Geometry: final body of the model. Coordinates: model frame, mm. A direction names the side the tool comes from. Coordinates: 2 decimals unless noted, no trailing zeros. Order: outer loops, then holes, each group sorted by start corner. A loop starts at its lowest first (then second) coordinate and runs counter-clockwise, first axis right, second up. Notation, with made-up numbers: M -0.5,-33 L 43.5,-33 A28 cw 43.5,-9 Z; hole C 50.5,64 d8. An arc over 180 degrees is marked long. Use CSV: the item, a comma, the result in double quotes. Start each with the question number.
Q1. Section query A-A, the plane y = 1.4. Output: boundary loops of the cut face in (x, z).
Q2. Ray query, probe 1 along X at (y, z) = (0.1, 3.75); probe 2 along Z at (x, y) = (6.5, 0.7); probe 3 along Z at (x, y) = (9.75, 0.3). Return the intervals inside material, ascending.
Q3. Access query for faces 1 (the face through (4, 1.6, -1)), 2 (the face through (3.5, 1, 3)). Directions: +Z, -Z, +X, -X, +Y, -Y. A direction counts if a zero-diameter tool reaches every point of the face in a straight line with its end or side. Return the directions, or none.
Q4. Mould query, pull axis X, two halves, no side actions, for faces 3 (the face through (9.53, 0.81, -0.75)), 4 (the face through (12.881, 0.811, 0.123)), 5 (the face through (-3.5, 1, 1)). Classes: +X half, -X half, draft (parallel to the pull), parting line (faces both ways), or undercut.
Q5. Section query D-D, the plane z = 1.75. Output: boundary loops of the cut face in (x, y), and give its area (3 significant figures).
Q6. Section query B-B, the plane z = 0.5. Output: boundary loops of the cut face in (x, y), and give its area (3 significant figures).
Q7. First-contact query: P1, Ø0.8, axis at x = 5, y = 1, coming from the +Z side. Flat tip, straight axial feed; report the tip coordinate or a pass-through.
Q8. Section query C-C, the plane x = 9.5. Output: boundary loops of the cut face in (y, z), and give its area (3 significant figures).
from build123d import *

# Parameters (mm, degrees)
ESBO_O2_W                = 12
ESBO_O2_H                = 5
RESSALTO_EXTRUS_O1_DEPTH = 1.6
ESBO_O3_R                = 1.5
CORTE_EXTRUS_O1_DEPTH    = 1.6
CORTE_EXTRUS_O2_DEPTH    = 1.6
FILETE1_R                = 1
FILETE2_R                = 1
FILETE6_R                = 0.5


with BuildPart() as part:
    # Esboço2 → Ressalto-extrusão1 (new body)
    with BuildSketch(Plane(origin=(0, 0, 0), x_dir=(1, 0, 0), z_dir=(0, 1, 0))):
        with BuildLine():
            Line((-3.5, 2.25), (-3.5, -4.25))
            Line((-3.5, -4.25), (3.5, -4.25))
            Line((3.5, -4.25), (3.5, -0.75))
            Line((3.5, -0.75), (3.5, 4.25))
            Line((3.5, 4.25), (-1.5, 4.25))
            ThreePointArc((-1.5, 4.25), (-2.914213562, 3.664213562), (-3.5, 2.25))
        make_face()
        with Locations((9.5, 1.75)):
            Rectangle(ESBO_O2_W, ESBO_O2_H)
    extrude(amount=RESSALTO_EXTRUS_O1_DEPTH)

    # Esboço3 → Corte-extrusão1 (cut)
    with BuildSketch(Plane(origin=(0, 1.6, 0), x_dir=(1, 0, 0), z_dir=(0, 1, 0))):
        with Locations((9.5, -0.75)):
            Circle(ESBO_O3_R)
    extrude(amount=-CORTE_EXTRUS_O1_DEPTH, mode=Mode.SUBTRACT)

    # Esboço4 → Corte-extrusão2 (cut)
    with BuildSketch(Plane(origin=(0, 1.6, 0), x_dir=(1, 0, 0), z_dir=(0, 1, 0))):
        Polygon((11, -0.75), (15.5, 0.75), (15.5, -0.75), align=None)
    extrude(amount=-CORTE_EXTRUS_O2_DEPTH, mode=Mode.SUBTRACT)

    # Filete1
    filete1_edges = [part.edges().sort_by_distance(p)[0] for p in [
        (15.5, 0.8, -0.75),
    ]]
    fillet(filete1_edges, radius=FILETE1_R)

    # Filete2
    filete2_edges = [part.edges().sort_by_distance(p)[0] for p in [
        (15.5, 0.8, -4.25),
    ]]
    fillet(filete2_edges, radius=FILETE2_R)

    # Filete6
    filete6_edges = [part.edges().sort_by_distance(p)[0] for p in [
        (3.5, 0.8, 0.75),
    ]]
    fillet(filete6_edges, radius=FILETE6_R)


solid = part.part
Responses:
1,outline,"M -3.5,-2.25 A2 ccw -1.5,-4.25 L 14.5,-4.25 A1 ccw 15.5,-3.25 L 15.5,-1.47 A1 ccw 14.82,-0.52 L 11,0.75 A1.5 cw 8,0.75 L 4,0.75 A0.5 cw 3.5,1.25 L 3.5,4.25 L -3.5,4.25 Z"
2,probe 1,"x = -3.5 to 3.5"
2,probe 2,"z = -4.25 to 0.75"
2,probe 3,"z = -4.25 to -0.73"
3,face 1,"+Z, -Z, +X, -X, +Y"
3,face 2,"+Z, +X, +Y, -Y"
4,face 3,"undercut"
4,face 4,"+X half"
4,face 5,"-X half"
5,outline,"M -3.5,0 L 3.5,0 L 3.5,1.6 L -3.5,1.6 Z"
5,area,"11.2 mm²"
6,outline,"M -3.5,0 L 8.02,0 L 8.02,1.6 L -3.5,1.6 Z; M 10.98,0 L 11.75,0 L 11.75,1.6 L 10.98,1.6 Z"
6,area,"19.7 mm²"
7,P1,"stops at z = 0.75"
8,outline,"M 0,-4.25 L 1.6,-4.25 L 1.6,-0.75 L 0,-0.75 Z"
8,area,"5.60 mm²"
